Print and shaded views of the part. All mm, measured from the part's lowest x, y and z. A direction names the side the tool comes from. Round coordinates to 2 decimals unless told otherwise and drop trailing zeros. Loops run counter-clockwise (first coordinate to the right, second up) from the corner with the lowest first, then second, coordinate; pieces in that order, holes last. Notation, with made-up numbers: (77.25, 85.5) - (120.25, 85.5) arc R20 cw to (120.25, 120.5) - close; hole circle Ø11 at (-8, 53). An arc over 180 degrees is marked (long way). Use one line per item in the form item = value.
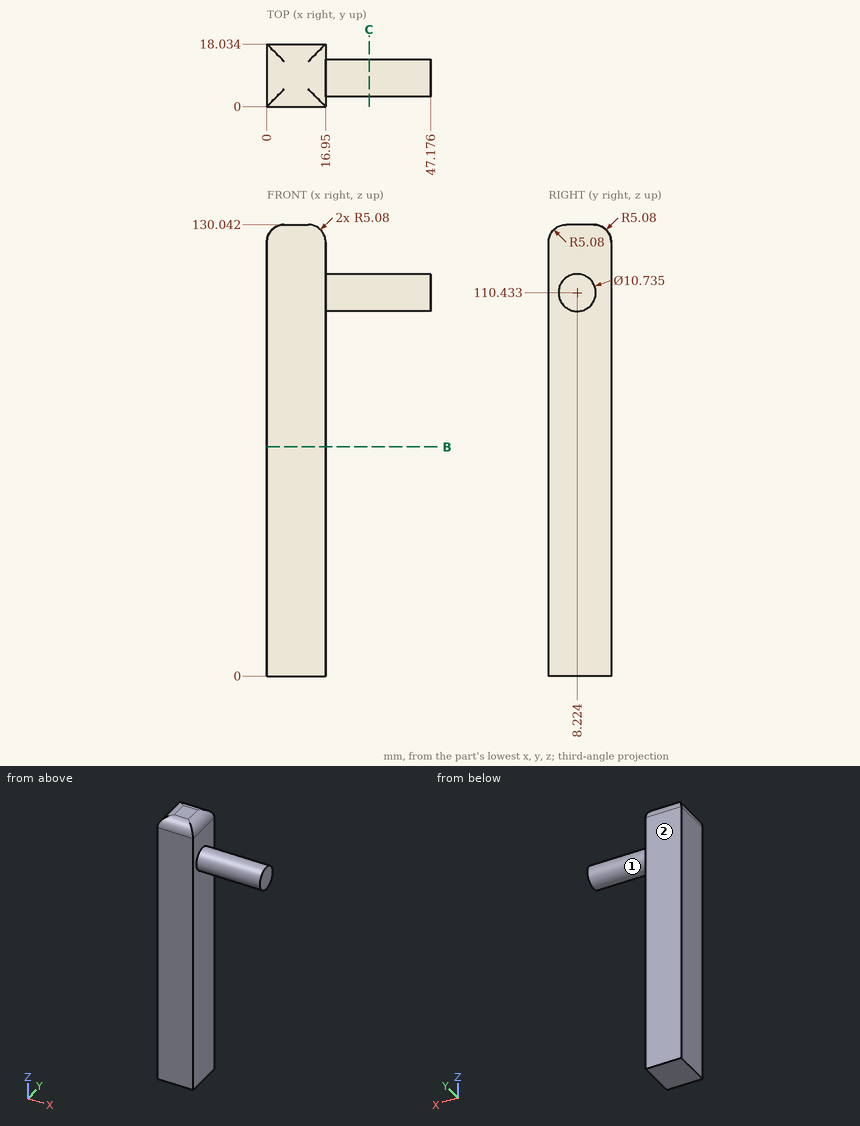
1) Tool access for the marked faces 1 and 2: list every direction of +Z, -Z, +X, -X, +Y, -Y with a clear straight run to the whole face (end or side of a thin tool).
Report:
face_1 = +X
face_2 = +Z, -Z, +X, -X, +Y
2) Slice it at B-B (z = 66). Write the cut outline in (x, y), plus the area to 3 significant figures.
Report:
outline = (0, 0) - (16.95, 0) - (16.95, 18.03) - (0, 18.03) - close
area = 306 mm^2
3) Slice it at C-C (x = 29.5). Write the cut outline in (y, z) (1 decimal), plus the area to 3 significant figures.
Report:
outline = circle Ø10.7 at (8.2, 110.4)
area = 90.5 mm^2
4) Flat gauge pins, fed straight in: pin 1 (2 mm diameter, centred on x = 24, y = 16, fed in from +Z); pin 2 (4 mm diameter, centred on x = 38.5, y = 15, fed in from +Z) (1 decimal); pin 3 (5.5 mm diameter, centred on y = 9, z = 76.5, fed in from +X). Where does each tip first touch, or does it go through?
Report:
pin_1 = through
pin_2 = 112.9
pin_3 = 16.95
5) Drill centre lines: probe 1 along X at (y, z) = (12.75, 81); probe 2 along Z at (x, y) = (44, 3.75) (1 decimal); probe 3 along Z at (x, y) = (8.5, 13.75). Where is each one in solid material? Low to high.
Report:
probe_1 = 0 to 16.95
probe_2 = 107.5 to 113.4
probe_3 = 0 to 129.98
